Read the model definition and answer for the solid it produces. Units are mm, in the model's axes. Face numbers are marked on the shaded views. A direction names the side the tool comes from. Coordinates: 2 decimals unless noted, no trailing zeros. Write each loop counter-clockwise with the first axis right and the second up, starting at its lowest first coordinate (ties: lowest second). Pieces come first, ordered by that corner, then holes. Notation, with made-up numbers: (-5.5, 6) -> (45.5, 6) arc R8 ccw to (45.5, 19) -> close; hole circle Ø2 at (-12.5, 62). An arc over 180 degrees is marked (long way). Answer in a Markdown table with one row per item. Add a question column.
Item 1: For a pull along X with two mould halves and no side action, classify the marked faces 3, 4 and 5 as +X half, -X half, draft (parallel to the pull), parting line (faces both ways), or undercut.
Item 2: Given pin 1 Ø4 at (x, y) = (-20.5, -13.5) entering from +Z; pin 2 Ø1 at (x, z) = (35.5, 12.5) entering from -Y; pin 3 Ø22 at (x, z) = (62, 28) entering from -Y; pin 4 Ø4 at (x, z) = (-4, 25.5) entering from -Y, each flat-ended and moving along its own axis, determine where each tip first touches the part or whether it passes through.
Item 3: Section C-C on z = 27 is taken. Write down the section's boundary in (x, y).
Item 4: Section A-A on y = -8.5 is taken. Write down the section's boundary in (x, z), then the cut area to 3 significant figures.
Item 5: Straight lines are drawn through the part: line 1 (Y direction, x = -1.5, z = -6.5); line 2 (X direction, y = -11.5, z = 57); line 3 (Y direction, x = -19, z = 60.5). For each, find the intervals that lie inside material, in ascending order. Write a range as from..to.
Item 6: Section D-D on x = 55.5 is taken. Write down the section's boundary in (y, z), then the cut area to 3 significant figures.
Item 7: Section B-B on x = 32 is taken. Write down the section's boundary in (y, z).
Item 8: Which of the six approach directions +Z, -Z, +X, -X, +Y, -Y give full straight-line access (tool end or side, diameter ignored) to the marked faces 1 and 2?
```python
from build123d import *

# Parameters (mm, degrees)
F1_DEPTH = 69.85


with BuildPart() as f1:
    # F0 (on Top) → F1 (new body, symmetric)
    with BuildSketch(Plane.XY):
        with BuildLine():
            Line((-70, 0), (-50, 0))
            ThreePointArc((-50, 0), (0, -21.010205), (50, 0))
            Line((50, 0), (70, 0))
            Line((70, 0), (70, 2))
            Line((70, 2), (-70, 2))
            Line((-70, 2), (-70, 0))
        make_face()
        with BuildLine():
            ThreePointArc((47.159304, 0), (0, -19.58378), (-47.159304, 0))
            Line((-47.159304, 0), (47.159304, 0))
        make_face(mode=Mode.SUBTRACT)
    extrude(amount=F1_DEPTH, both=True)


solid = f1.part
```
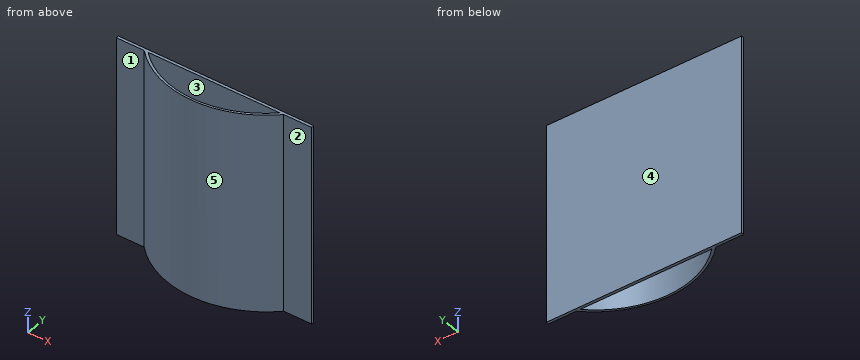
Results below:
| question | item | result |
|---|---|---|
| 1 | face 3 | undercut |
| 1 | face 4 | draft |
| 1 | face 5 | parting line |
| 2 | pin 1 | passes through |
| 2 | pin 2 | stops at y = -11.63 |
| 2 | pin 3 | stops at y = 0 |
| 2 | pin 4 | stops at y = -20.98 |
| 3 | outline | (-70, 0) -> (-50, 0) arc R70 ccw to (50, 0) -> (70, 0) -> (70, 2) -> (-70, 2) -> close; hole (-47.16, 0) arc R66.57 ccw to (47.16, 0) -> close |
| 4 | outline | (-39.94, -69.85) -> (-36.78, -69.85) -> (-36.78, 69.85) -> (-39.94, 69.85) -> close; (36.78, -69.85) -> (39.94, -69.85) -> (39.94, 69.85) -> (36.78, 69.85) -> close |
| 4 | area | 881 mm2 |
| 5 | line 1 | y = -20.99..-19.57, 0..2 |
| 5 | line 2 | x = -35.23..-31.8, 31.8..35.23 |
| 5 | line 3 | y = -18.38..-16.81, 0..2 |
| 6 | outline | (0, -69.85) -> (2, -69.85) -> (2, 69.85) -> (0, 69.85) -> close |
| 6 | area | 279 mm2 |
| 7 | outline | (-13.27, -69.85) -> (-11.39, -69.85) -> (-11.39, 69.85) -> (-13.27, 69.85) -> close; (0, -69.85) -> (2, -69.85) -> (2, 69.85) -> (0, 69.85) -> close |
| 8 | face 1 | +Z, -Z, -X, -Y |
| 8 | face 2 | +Z, -Z, +X, -Y |
